Could you check a few things on this model? Use its own coordinates, in mm. Face numbers are marked on the shaded views. Coordinates: 2 decimals unless noted, no trailing zeros. Loops run counter-clockwise (first coordinate to the right, second up) from the corner with the lowest first, then second, coordinate; pieces in that order, holes last. Notation, with made-up numbers: (67.5, 68) - (96.5, 68) arc R20 ccw to (96.5, 93) - close; hole circle Ø3 at (33, 66.5). An arc over 180 degrees is marked (long way). One line per item, written item: value. Start each with the question number.
(1) If we section it at C-C on x = 31.5: Write out the boundary of the cut face in (y, z), then the cut area to 3 significant figures.
(2) If I drill on line 1 along X through (y, z) = (-28.5, 24.25); line 2 along Y through (x, z) = (-12, 21.75); line 3 along Y through (x, z) = (35.05, 21.15), over which ranges is the centre line in solid material (lowest first)? Write a range as from..to.
(3) If we section it at A-A on z = 21.15: Write out the boundary of the cut face in (x, y), then the cut area to 3 significant figures.
(4) I'm going to push flat-ended pins straight in: P1, Ø11.5, axis at x = 7.5, y = -7.5, coming from the -Z side; P2, Ø1, axis at x = -5.5, y = -28, coming from the -Z side. Where does each tip first touch, or does it pass through?
(5) If we mould it in two halves opening along X, with no side actions, what happens to the marked faces 1, 2, 3 and 4? For each: pulls with the +X half, pulls with the -X half, needs draft (parallel to the pull), parting line crosses it, or undercut.
(6) If we section it at B-B on y = 2.5: Write out the boundary of the cut face in (x, z).
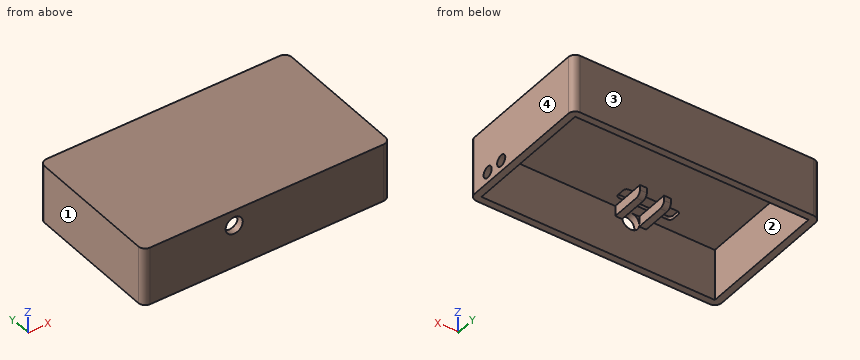
```python
from build123d import *

# Parameters (mm, degrees)
BOX017_W          = 16
BOX017_H          = 4
BOX017_DEPTH      = 1
FILLET004_R       = 1
CYLINDER025_R     = 1.65
CYLINDER025_DEPTH = 10
CYLINDER024_R     = 1.65
CYLINDER024_DEPTH = 10
BOX015_W          = 2
BOX015_H          = 10
BOX015_DEPTH      = 5
FILLET006_R       = 1.5
CYLINDER023_R     = 2.5
CYLINDER023_DEPTH = 2
BOX009_W          = 68
BOX009_H          = 38
BOX009_DEPTH      = 15
BOX008_W          = 72
BOX008_H          = 42
BOX008_DEPTH      = 17
FILLET_R          = 2
BOX018_W          = 2
BOX018_H          = 10
BOX018_DEPTH      = 5
FILLET005_R       = 1.5


with BuildPart() as fillet004:
    # Box017 → Box017 (new body)
    with BuildSketch(Plane(origin=(-19, -30.6, 33), x_dir=(1, 0, 0), z_dir=(0, 0, 1))):
        with Locations((8, 2)):
            Rectangle(BOX017_W, BOX017_H)
    extrude(amount=BOX017_DEPTH)

    # Fillet004
    fillet004_edges = [fillet004.edges().sort_by_distance(p)[0] for p in [
        (-19, -30.6, 33.5),
        (-19, -26.6, 33.5),
        (-3, -30.6, 33.5),
        (-3, -26.6, 33.5),
    ]]
    fillet(fillet004_edges, radius=FILLET004_R)


with BuildPart() as cylinder025:
    # Cylinder025 → Cylinder025 (new body)
    with BuildSketch(Plane(origin=(33.99, -22.8034, 21.15), x_dir=(0, 0, -1), z_dir=(1, 0, 0))):
        Circle(CYLINDER025_R)
    extrude(amount=CYLINDER025_DEPTH)


with BuildPart() as fusion018:
    # Cylinder024 → Cylinder024 (new body)
    with BuildSketch(Plane(origin=(33.99, -28.3034, 21.15), x_dir=(0, 0, -1), z_dir=(1, 0, 0))):
        Circle(CYLINDER024_R)
    extrude(amount=CYLINDER024_DEPTH)

    # Fusion018: union Cylinder025
    add(cylinder025.part)


with BuildPart() as fillet006:
    # Box015 → Box015 (new body)
    with BuildSketch(Plane(origin=(-14, -33.6, 30), x_dir=(1, 0, 0), z_dir=(0, 0, 1))):
        with Locations((1, 5)):
            Rectangle(BOX015_W, BOX015_H)
    extrude(amount=BOX015_DEPTH)

    # Fillet006
    fillet006_edges = [fillet006.edges().sort_by_distance(p)[0] for p in [
        (-13, -23.6, 30),
    ]]
    fillet(fillet006_edges, radius=FILLET006_R)


with BuildPart() as cylinder023:
    # Cylinder023 → Cylinder023 (new body)
    with BuildSketch(Plane(origin=(-9.5, -33.6034, 30.5), x_dir=(1, 0, 0), z_dir=(0, -1, 0))):
        Circle(CYLINDER023_R)
    extrude(amount=CYLINDER023_DEPTH)


with BuildPart() as kostka009:
    # Box009 → Box009 (new body)
    with BuildSketch(Plane(origin=(-34.01, -33.6034, 18), x_dir=(1, 0, 0), z_dir=(0, 0, 1))):
        with Locations((34, 19)):
            Rectangle(BOX009_W, BOX009_H)
    extrude(amount=BOX009_DEPTH)


with BuildPart() as cut020:
    # Box008 → Box008 (new body)
    with BuildSketch(Plane(origin=(-36.01, -35.6034, 18), x_dir=(1, 0, 0), z_dir=(0, 0, 1))):
        with Locations((36, 21)):
            Rectangle(BOX008_W, BOX008_H)
    extrude(amount=BOX008_DEPTH)

    # Cut005: cut Kostka009
    add(kostka009.part, mode=Mode.SUBTRACT)

    # Fillet
    fillet_edges = [cut020.edges().sort_by_distance(p)[0] for p in [
        (-36.01, -35.6034, 26.5),
        (-36.01, 6.3966, 26.5),
        (35.99, -35.6034, 26.5),
        (35.99, 6.3966, 26.5),
    ]]
    fillet(fillet_edges, radius=FILLET_R)

    # Cut020: cut Cylinder023
    add(cylinder023.part, mode=Mode.SUBTRACT)


with BuildPart() as cover:
    # Box018 → Box018 (new body)
    with BuildSketch(Plane(origin=(-7, -33.6, 30), x_dir=(1, 0, 0), z_dir=(0, 0, 1))):
        with Locations((1, 5)):
            Rectangle(BOX018_W, BOX018_H)
    extrude(amount=BOX018_DEPTH)

    # Fillet005
    fillet005_edges = [cover.edges().sort_by_distance(p)[0] for p in [
        (-6, -23.6, 30),
    ]]
    fillet(fillet005_edges, radius=FILLET005_R)

    # Fusion017: union Fillet006, Cut020
    add(fillet006.part)
    add(cut020.part)

    # Cut021: cut Fusion018
    add(fusion018.part, mode=Mode.SUBTRACT)

    # Cut022: cut Fillet004
    add(fillet004.part, mode=Mode.SUBTRACT)


solid = cover.part
```
Values:
1. outline: (-35.6, 18) - (-33.6, 18) - (-33.6, 33) - (4.4, 33) - (4.4, 18) - (6.4, 18) - (6.4, 35) - (-35.6, 35) - close
1. area: 144 mm2
2. line 1: x = -36.01..-34.01, 33.99..35.99
2. line 2: y = -35.6..-33.6, 4.4..6.4
2. line 3: y = -35.3..-29.95, -26.65..-24.45, -21.15..6.09
3. outline: (-36.01, -33.6) arc R2 ccw to (-34.01, -35.6) - (33.99, -35.6) arc R2 ccw to (35.99, -33.6) - (35.99, -29.95) - (33.99, -29.95) - (33.99, -33.6) - (-34.01, -33.6) - (-34.01, 4.4) - (33.99, 4.4) - (33.99, -21.15) - (35.99, -21.15) - (35.99, 4.4) arc R2 ccw to (33.99, 6.4) - (-34.01, 6.4) arc R2 ccw to (-36.01, 4.4) - close; (33.99, -26.65) - (35.99, -26.65) - (35.99, -24.45) - (33.99, -24.45) - close
3. area: 423 mm2
4. P1: stops at z = 33
4. P2: stops at z = 30
5. face 1: pulls with the -X half
5. face 2: undercut
5. face 3: needs draft
5. face 4: pulls with the +X half
6. outline: (-36.01, 18) - (-34.01, 18) - (-34.01, 33) - (33.99, 33) - (33.99, 18) - (35.99, 18) - (35.99, 35) - (-36.01, 35) - close
